Geometry check sheet. Reference: the model listing, model coordinates, mm. Round coordinates to 2 decimals unless told otherwise and drop trailing zeros. Order: outer loops, then holes, each group sorted by start corner. A loop starts at its lowest first (then second) coordinate and runs counter-clockwise, first axis right, second up. Notation, with made-up numbers: (32.5, -37) - (82.5, -37) arc R17 cw to (82.5, -25) - close; hole circle Ø4 at (-31, 40.25). An arc over 180 degrees is marked (long way). Return JSON: item names as keys, results as strings. Group by question number.
Q1. Sectioned sample at D-D, the plane y = 33. Record the cut outline in (x, z), then the cut area to 3 significant figures.
Q2. Material ranges on line 1 along X through (y, z) = (-28, 0.25); line 2 along X through (y, z) = (21, -0.2); line 3 along Y through (x, z) = (-30, 0.1), recorded low to high.
Q3. Sectioned sample at B-B, the plane z = -0.1. Record the cut outline in (x, y).
Q4. Sectioned sample at A-A, the plane x = 4.5. Record the cut outline in (y, z), then the cut area to 3 significant figures.
Q5. Sectioned sample at C-C, the plane y = 14. Record the cut outline in (x, z).
```python
from build123d import *

# Parameters (mm, degrees)
ESQUISSE1_R          = 2.1
BASE_EXTRUSION_DEPTH = 0.3


with BuildPart() as part:
    # Esquisse1 → Base-Extrusion (new, symmetric)
    with BuildSketch(Plane.XY):
        with BuildLine():
            Line((35.615327088, -25.672223926), (33.690495331, -5.355736059))
            ThreePointArc((33.690495331, -5.355736059), (32.627582421, 0.138570374), (30.529161577, 5.326423206))
            Line((30.529161577, 5.326423206), (20.291189648, 24.943575231))
            ThreePointArc((20.291189648, 24.943575231), (19.367522251, 26.19363098), (18.105897834, 27.101433088))
            Line((18.105897834, 27.101433088), (1.120998661, 35.694422442))
            ThreePointArc((1.120998661, 35.694422442), (-9.646140892, 36.898255889), (-18.57139047, 30.756559943))
            Line((-18.57139047, 30.756559943), (-21.986449586, 26.007166333))
            Line((-21.986449586, 26.007166333), (-33.307069298, 21.886797725))
            ThreePointArc((-33.307069298, 21.886797725), (-35.52580407, 20.184302655), (-36.366774139, 17.517086354))
            Line((-36.366774139, 17.517086354), (-36.366774139, 5.469934486))
            Line((-36.366774139, 5.469934486), (-39.661725259, 0.636440352))
            ThreePointArc((-39.661725259, 0.636440352), (-42.380416479, -9.851134542), (-37.566604459, -19.557200839))
            Line((-37.566604459, -19.557200839), (-23.682658123, -32.578809807))
            ThreePointArc((-23.682658123, -32.578809807), (-22.398102217, -33.453862354), (-20.907521199, -33.894281545))
            Line((-20.907521199, -33.894281545), (1.028164427, -36.805367071))
            ThreePointArc((1.028164427, -36.805367071), (6.620853648, -37.002887485), (12.147350486, -36.122535429))
            Line((12.147350486, -36.122535429), (31.896935448, -30.982637535))
            ThreePointArc((31.896935448, -30.982637535), (34.733377642, -29.011706008), (35.615327088, -25.672223926))
        make_face()
        with Locations((15.838548739, 22.619791811)):
            Circle(ESQUISSE1_R, mode=Mode.SUBTRACT)
        with Locations((-31.716624427, 17.517086354)):
            Circle(ESQUISSE1_R, mode=Mode.SUBTRACT)
        with Locations((-20.246771948, -28.915387001)):
            Circle(ESQUISSE1_R, mode=Mode.SUBTRACT)
        with Locations((30.63761742, -26.143823826)):
            Circle(ESQUISSE1_R, mode=Mode.SUBTRACT)
        with BuildLine():
            Line((-34.768380459, -1.709606371), (-14.693205187, 26.96071518))
            ThreePointArc((-14.693205187, 26.96071518), (-8.23816652, 31.073028346), (-0.76592038, 29.416471259))
            Line((-0.76592038, 29.416471259), (13.569240395, 19.378883623))
            ThreePointArc((13.569240395, 19.378883623), (20.322569613, -18.921149595), (-17.977463605, -25.674478813))
            Line((-17.977463605, -25.674478813), (-32.31262438, -15.636891177))
            ThreePointArc((-32.31262438, -15.636891177), (-36.424937546, -9.181852511), (-34.768380459, -1.709606371))
        make_face(mode=Mode.SUBTRACT)
    extrude(amount=BASE_EXTRUSION_DEPTH, both=True)


solid = part.part
```
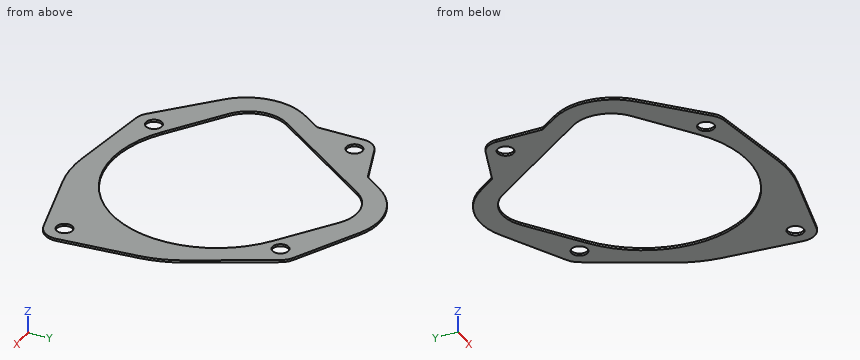
Reply:
{
 "1": {"outline": "(-16.66, -0.3) - (6.45, -0.3) - (6.45, 0.3) - (-16.66, 0.3) - close", "area": "13.9 mm^2"},
 "2": {"line 1": "-28.56 to -22.14, -18.36 to -13.98, 9.57 to 29.66, 31.62 to 35.28", "line 2": "-34.8 to -18.87, 11.25 to 14.5, 17.18 to 22.35", "line 3": "-26.65 to -17.26, 5.1 to 16.31, 18.73 to 23.09"},
 "3": {"outline": "(-39.66, 0.64) arc R15.5 ccw to (-37.57, -19.56) - (-23.68, -32.58) arc R5.02 ccw to (-20.91, -33.89) - (1.03, -36.81) arc R29 ccw to (12.15, -36.12) - (31.9, -30.98) arc R5 ccw to (35.62, -25.67) - (33.69, -5.36) arc R29 ccw to (30.53, 5.33) - (20.29, 24.94) arc R5.02 ccw to (18.11, 27.1) - (1.12, 35.69) arc R15.5 ccw to (-18.57, 30.76) - (-21.99, 26.01) - (-33.31, 21.89) arc R4.65 ccw to (-36.37, 17.52) - (-36.37, 5.47) - close; hole (-34.77, -1.71) arc R10 ccw to (-32.31, -15.64) - (-17.98, -25.67) arc R27.5 ccw to (13.57, 19.38) - (-0.77, 29.42) arc R10 ccw to (-14.69, 26.96) - close; hole circle Ø4.2 at (-31.72, 17.52); hole circle Ø4.2 at (-20.25, -28.92); hole circle Ø4.2 at (15.84, 22.62); hole circle Ø4.2 at (30.64, -26.14)"},
 "4": {"outline": "(-37.06, -0.3) - (-29.82, -0.3) - (-29.82, 0.3) - (-37.06, 0.3) - close; (25.73, -0.3) - (33.98, -0.3) - (33.98, 0.3) - (25.73, 0.3) - close", "area": "9.30 mm^2"},
 "5": {"outline": "(-36.37, -0.3) - (-23.77, -0.3) - (-23.77, 0.3) - (-36.37, 0.3) - close; (19.29, -0.3) - (26, -0.3) - (26, 0.3) - (19.29, 0.3) - close"}
}
